Verification items for the finished model (mm, model axes). A direction names the side the tool comes from. Round coordinates to 2 decimals unless told otherwise and drop trailing zeros. Write each loop counter-clockwise with the first axis right and the second up, starting at its lowest first coordinate (ties: lowest second). Pieces come first, ordered by that corner, then holes. Notation, with made-up numbers: (-9, -35.75) - (39, -35.75) arc R18 ccw to (39, -24.75) - close; hole circle Ø10 at (75.5, 10.25). An arc over 180 degrees is marked (long way). Answer as a JSON object with one key per item and string values.
```python
from build123d import *

# Parameters (mm, degrees)
CYLINDER002001001002002001002_R           = 1
CYLINDER002001001002002001002_DEPTH       = 40
CYLINDER002001001002002001002001003_R     = 1.5
CYLINDER002001001002002001002001003_DEPTH = 40
CYLINDER002001001002002001002001002_R     = 1.5
CYLINDER002001001002002001002001002_DEPTH = 40
CYLINDER002001001002002001002001001_R     = 1.5
CYLINDER002001001002002001002001001_DEPTH = 40
CYLINDER002001001002002001002001_R        = 1
CYLINDER002001001002002001002001_DEPTH    = 40
CYLINDER002001001002002001001_R           = 12
CYLINDER002001001002002001001_DEPTH       = 26
CYLINDER002001001002002001001_PITCH_ANGLE = 90
CYLINDER001001001_R                       = 12
CYLINDER001001001_DEPTH                   = 26
CYLINDER001001001_PITCH_ANGLE             = 90
BOX001002001003002001001001001001_W       = 40
BOX001002001003002001001001001001_H       = 10
BOX001002001003002001001001001001_DEPTH   = 3
BOX001002001003002001001001001_W          = 40
BOX001002001003002001001001001_H          = 12
BOX001002001003002001001001001_DEPTH      = 3
BOX001002001003002001001001_W             = 40
BOX001002001003002001001001_H             = 10
BOX001002001003002001001001_DEPTH         = 3
BOX001002001003002001003_W                = 10
BOX001002001003002001003_H                = 12
BOX001002001003002001003_DEPTH            = 4
CYLINDER002001001002003001_R              = 6
CYLINDER002001001002003001_DEPTH          = 4
BOX001002001003002001002_W                = 26
BOX001002001003002001002_H                = 40
BOX001002001003002001002_DEPTH            = 24
CYLINDER001001_R                          = 14
CYLINDER001001_DEPTH                      = 26
CYLINDER001001_PITCH_ANGLE                = 90
CYLINDER002001001002002001_R              = 14
CYLINDER002001001002002001_DEPTH          = 26
CYLINDER002001001002002001_PITCH_ANGLE    = 90
BOX001002001003002001001_W                = 40
BOX001002001003002001001_H                = 40
BOX001002001003002001001_DEPTH            = 5
BOX001002001003002001_W                   = 26
BOX001002001003002001_H                   = 40
BOX001002001003002001_DEPTH               = 28


with BuildPart() as cylinder006:
    # Cylinder002001001002002001002 → Cylinder002001001002002001002 (new body)
    with BuildSketch(Plane(origin=(74, 42.5, 0), x_dir=(1, 0, 0), z_dir=(0, 0, 1))):
        Circle(CYLINDER002001001002002001002_R)
    extrude(amount=CYLINDER002001001002002001002_DEPTH)


with BuildPart() as cylinder0010:
    # Cylinder002001001002002001002001003 → Cylinder002001001002002001002001003 (new body)
    with BuildSketch(Plane(origin=(99, 15, 0), x_dir=(1, 0, 0), z_dir=(0, 0, 1))):
        Circle(CYLINDER002001001002002001002001003_R)
    extrude(amount=CYLINDER002001001002002001002001003_DEPTH)


with BuildPart() as cylinder009:
    # Cylinder002001001002002001002001002 → Cylinder002001001002002001002001002 (new body)
    with BuildSketch(Plane(origin=(99, 45.5, 0), x_dir=(1, 0, 0), z_dir=(0, 0, 1))):
        Circle(CYLINDER002001001002002001002001002_R)
    extrude(amount=CYLINDER002001001002002001002001002_DEPTH)


with BuildPart() as cylinder008:
    # Cylinder002001001002002001002001001 → Cylinder002001001002002001002001001 (new body)
    with BuildSketch(Plane(origin=(84, 30, 0), x_dir=(1, 0, 0), z_dir=(0, 0, 1))):
        Circle(CYLINDER002001001002002001002001001_R)
    extrude(amount=CYLINDER002001001002002001002001001_DEPTH)


with BuildPart() as batteryframeholes:
    # Cylinder002001001002002001002001 → Cylinder002001001002002001002001 (new body)
    with BuildSketch(Plane(origin=(74, 17.5, 0), x_dir=(1, 0, 0), z_dir=(0, 0, 1))):
        Circle(CYLINDER002001001002002001002001_R)
    extrude(amount=CYLINDER002001001002002001002001_DEPTH)

    # Fusion002001002002002001005: union Cylinder006, Cylinder0010, Cylinder009, Cylinder008
    add(cylinder006.part)
    add(cylinder0010.part)
    add(cylinder009.part)
    add(cylinder008.part)


with BuildPart() as cylinder005:
    # Cylinder002001001002002001001 → Cylinder002001001002002001001 (new body)
    with BuildSketch(Plane.XY):
        Circle(CYLINDER002001001002002001001_R)
    extrude(amount=CYLINDER002001001002002001001_DEPTH)


with BuildPart() as cylinder005_1:
    # Cylinder002001001002002001001 pitch: moved
    add(cylinder005.part.rotate(Axis((0, 0, 0), (0, 1, 0)), CYLINDER002001001002002001001_PITCH_ANGLE))


with BuildPart() as cylinder005_2:
    # Cylinder002001001002002001001 placement: moved
    add(cylinder005_1.part.moved(Location((2, 10, 19))))


with BuildPart() as cylinder004:
    # Cylinder001001001 → Cylinder001001001 (new body)
    with BuildSketch(Plane.XY):
        Circle(CYLINDER001001001_R)
    extrude(amount=CYLINDER001001001_DEPTH)


with BuildPart() as cylinder004_1:
    # Cylinder001001001 pitch: moved
    add(cylinder004.part.rotate(Axis((0, 0, 0), (0, 1, 0)), CYLINDER001001001_PITCH_ANGLE))


with BuildPart() as cylinder004_2:
    # Cylinder001001001 placement: moved
    add(cylinder004_1.part.moved(Location((2, 50, 19))))


with BuildPart() as box008:
    # Box001002001003002001001001001001 → Box001002001003002001001001001001 (new body)
    with BuildSketch(Plane(origin=(2, 38, 5), x_dir=(1, 0, 0), z_dir=(0, 0, 1))):
        with Locations((20, 5)):
            Rectangle(BOX001002001003002001001001001001_W, BOX001002001003002001001001001001_H)
    extrude(amount=BOX001002001003002001001001001001_DEPTH)


with BuildPart() as box007:
    # Box001002001003002001001001001 → Box001002001003002001001001001 (new body)
    with BuildSketch(Plane(origin=(2, 24, 5), x_dir=(1, 0, 0), z_dir=(0, 0, 1))):
        with Locations((20, 6)):
            Rectangle(BOX001002001003002001001001001_W, BOX001002001003002001001001001_H)
    extrude(amount=BOX001002001003002001001001001_DEPTH)


with BuildPart() as box006:
    # Box001002001003002001001001 → Box001002001003002001001001 (new body)
    with BuildSketch(Plane(origin=(2, 12, 5), x_dir=(1, 0, 0), z_dir=(0, 0, 1))):
        with Locations((20, 5)):
            Rectangle(BOX001002001003002001001001_W, BOX001002001003002001001001_H)
    extrude(amount=BOX001002001003002001001001_DEPTH)


with BuildPart() as box005:
    # Box001002001003002001003 → Box001002001003002001003 (new body)
    with BuildSketch(Plane(origin=(20, 24, 30), x_dir=(1, 0, 0), z_dir=(0, 0, 1))):
        with Locations((5, 6)):
            Rectangle(BOX001002001003002001003_W, BOX001002001003002001003_H)
    extrude(amount=BOX001002001003002001003_DEPTH)


with BuildPart() as powerbutton001:
    # Cylinder002001001002003001 → Cylinder002001001002003001 (new body)
    with BuildSketch(Plane(origin=(20, 30, 30), x_dir=(1, 0, 0), z_dir=(0, 0, 1))):
        Circle(CYLINDER002001001002003001_R)
    extrude(amount=CYLINDER002001001002003001_DEPTH)


with BuildPart() as fusion002001002002002001004:
    # Box001002001003002001002 → Box001002001003002001002 (new body)
    with BuildSketch(Plane(origin=(2, 10, 7), x_dir=(1, 0, 0), z_dir=(0, 0, 1))):
        with Locations((13, 20)):
            Rectangle(BOX001002001003002001002_W, BOX001002001003002001002_H)
    extrude(amount=BOX001002001003002001002_DEPTH)

    # Fusion002001002002002001004: union Cylinder005, Cylinder004, Box008, Box007, Box006, Box005, PowerButton001
    add(cylinder005_2.part)
    add(cylinder004_2.part)
    add(box008.part)
    add(box007.part)
    add(box006.part)
    add(box005.part)
    add(powerbutton001.part)


with BuildPart() as cylinder002:
    # Cylinder001001 → Cylinder001001 (new body)
    with BuildSketch(Plane.XY):
        Circle(CYLINDER001001_R)
    extrude(amount=CYLINDER001001_DEPTH)


with BuildPart() as cylinder002_1:
    # Cylinder001001 pitch: moved
    add(cylinder002.part.rotate(Axis((0, 0, 0), (0, 1, 0)), CYLINDER001001_PITCH_ANGLE))


with BuildPart() as cylinder002_2:
    # Cylinder001001 placement: moved
    add(cylinder002_1.part.moved(Location((0, 50, 19))))


with BuildPart() as cylinder003:
    # Cylinder002001001002002001 → Cylinder002001001002002001 (new body)
    with BuildSketch(Plane.XY):
        Circle(CYLINDER002001001002002001_R)
    extrude(amount=CYLINDER002001001002002001_DEPTH)


with BuildPart() as cylinder003_1:
    # Cylinder002001001002002001 pitch: moved
    add(cylinder003.part.rotate(Axis((0, 0, 0), (0, 1, 0)), CYLINDER002001001002002001_PITCH_ANGLE))


with BuildPart() as cylinder003_2:
    # Cylinder002001001002002001 placement: moved
    add(cylinder003_1.part.moved(Location((0, 10, 19))))


with BuildPart() as box003:
    # Box001002001003002001001 → Box001002001003002001001 (new body)
    with BuildSketch(Plane(origin=(0, 10, 2), x_dir=(1, 0, 0), z_dir=(0, 0, 1))):
        with Locations((20, 20)):
            Rectangle(BOX001002001003002001001_W, BOX001002001003002001001_H)
    extrude(amount=BOX001002001003002001001_DEPTH)


with BuildPart() as batteryframe2:
    # Box001002001003002001 → Box001002001003002001 (new body)
    with BuildSketch(Plane(origin=(0, 10, 5), x_dir=(1, 0, 0), z_dir=(0, 0, 1))):
        with Locations((13, 20)):
            Rectangle(BOX001002001003002001_W, BOX001002001003002001_H)
    extrude(amount=BOX001002001003002001_DEPTH)

    # Fusion002001002002002001003: union Cylinder002, Cylinder003, Box003
    add(cylinder002_2.part)
    add(cylinder003_2.part)
    add(box003.part)

    # Cut001: cut Fusion002001002002002001004
    add(fusion002001002002002001004.part, mode=Mode.SUBTRACT)


with BuildPart() as batteryframe2_1:
    # Cut001 placement: moved
    add(batteryframe2.part.moved(Location((67, 0, 0))))

    # Cut002: cut BatteryFrameHoles
    add(batteryframeholes.part, mode=Mode.SUBTRACT)


solid = batteryframe2_1.part
```
Q1. Release check for a two-part mould opening along Z. For faces 1 (the cylindrical face through (80, 64, 19)), 2 (the flat face through (88, 36, 6)), 3 (the flat face through (87, 30, 2)) record: released by +Z, released by -Z, zero draft, split by the parting line, or undercut.
Geometry check:
{"face 1": "split by the parting line", "face 2": "undercut", "face 3": "released by -Z"}
Q2. Material ranges on line 1 along Y through (x, z) = (99, 3.4); line 2 along X through (y, z) = (30, 4.35); line 3 along Y through (x, z) = (74, 31.8), recorded low to high. Write a range as [from, to].
Geometry check:
{"line 1": "y = [10, 13.5], [16.5, 44], [47, 50]", "line 2": "x = [67, 82.5], [85.5, 107]", "line 3": "y = [4.33, 16.5], [18.5, 41.5], [43.5, 55.67]"}
Q3. Section check A-A, the plane y = 42.5. Record the cut outline in (x, z).
Geometry check:
{"outline": "(67, 2) - (73, 2) - (73, 5) - (69, 5) - (69, 31) - (73, 31) - (73, 33) - (67, 33) - close; (75, 2) - (107, 2) - (107, 5) - (75, 5) - close; (75, 31) - (93, 31) - (93, 33) - (75, 33) - close"}
Q4. Set-up check for faces 4 (the flat face through (88, 43, 5)), 5 (the flat face through (91, 50, 4)), 6 (the flat face through (90, 24, 32)): record each of +Z, -Z, +X, -X, +Y, -Y from which the full face is reachable in a straight line by a thin tool's end or side.
Geometry check:
{"face 4": "+X", "face 5": "-Z, +X, +Y", "face 6": "+Z, +X"}
Q5. Gauge pin test, flat ends, axial feed: P1, Ø1, axis at x = 90.5, z = 32, coming from the -Y side; P2, Ø1, axis at x = 91.5, z = 23.5, coming from the -Y side; P3, Ø2, axis at x = 84, z = 20.5, coming from the -Y side; P4, Ø3, axis at y = 10, z = 8, coming from the +X side. Record the tip position at first contact, or that the pin passes through.
Geometry check:
{"P1": "stops at y = 3.7", "P2": "stops at y = -3.42", "P3": "stops at y = -3.99", "P4": "stops at x = 107"}
Q6. Section check C-C, the plane y = 15. Record the cut outline in (x, z), then the cut area to 3 significant figures.
Geometry check:
{"outline": "(67, 2) - (97.5, 2) - (97.5, 5) - (69, 5) - (69, 31) - (93, 31) - (93, 33) - (67, 33) - close; (100.5, 2) - (107, 2) - (107, 5) - (100.5, 5) - close", "area": "215 mm2"}
Q7. Section check D-D, the plane z = 4. Record the cut outline in (x, y).
Geometry check:
{"outline": "(67, 10) - (107, 10) - (107, 50) - (67, 50) - close; hole circle Ø2 at (74, 17.5); hole circle Ø2 at (74, 42.5); hole circle Ø3 at (84, 30); hole circle Ø3 at (99, 15); hole circle Ø3 at (99, 45.5)"}
Q8. Section check B-B, the plane x = 99. Record the cut outline in (y, z), then the cut area to 3 significant figures.
Geometry check:
{"outline": "(10, 2) - (13.5, 2) - (13.5, 5) - (12, 5) - (12, 7) - (10, 7) - close; (16.5, 2) - (44, 2) - (44, 5) - (38, 5) - (38, 7) - (36, 7) - (36, 5) - (24, 5) - (24, 7) - (22, 7) - (22, 5) - (16.5, 5) - close; (47, 2) - (50, 2) - (50, 7) - (48, 7) - (48, 5) - (47, 5) - close", "area": "118 mm2"}
